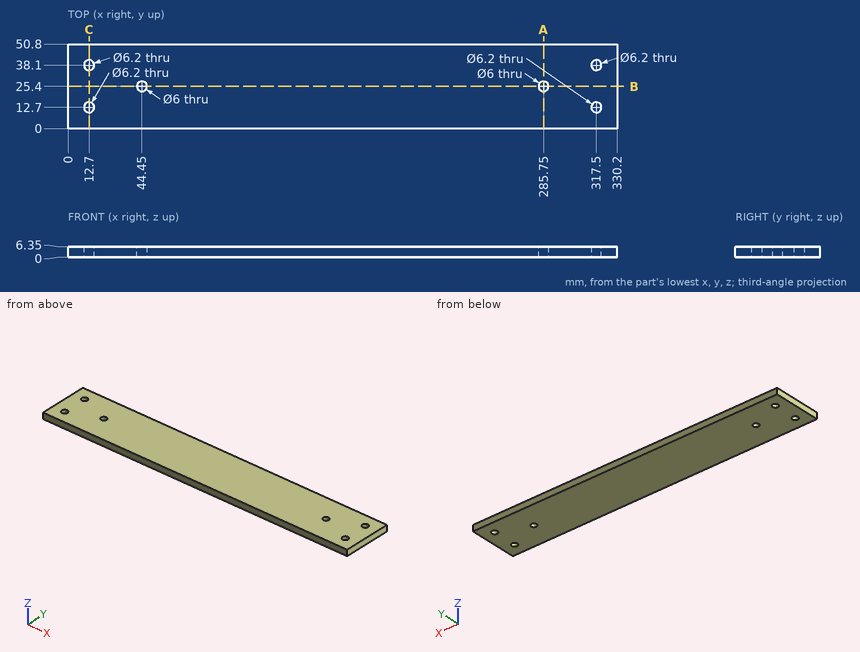
Input: dimensioned drawing with shaded views. Units: mm. Origin: part minimum x, y, z. Coordinates: 2 decimals unless noted, no trailing zeros. Order: outer loops, then holes, each group sorted by start corner. A loop starts at its lowest first (then second) coordinate and runs counter-clockwise, first axis right, second up.
Item 1: Section query C-C (x = 12.7). Output: boundary loops of the cut face in (y, z).
Answer:
outline: (0, 0) - (9.6, 0) - (9.6, 6.35) - (0, 6.35) - close; (15.8, 0) - (35, 0) - (35, 6.35) - (15.8, 6.35) - close; (41.2, 0) - (50.8, 0) - (50.8, 6.35) - (41.2, 6.35) - close
Item 2: Section query A-A (x = 285.75). Output: boundary loops of the cut face in (y, z), then the cut area to 3 significant figures.
Answer:
outline: (0, 0) - (22.4, 0) - (22.4, 6.35) - (0, 6.35) - close; (28.4, 0) - (50.8, 0) - (50.8, 6.35) - (28.4, 6.35) - close
area: 284 mm2
Item 3: Material intervals for line 1 along Y through (x, z) = (12.7, 3.5); line 2 along X through (y, z) = (10.5, 2.75); line 3 along X through (y, z) = (12, 4.75), sorted ascending.
Answer:
line 1: y = 0 to 9.6, 15.8 to 35, 41.2 to 50.8
line 2: x = 0 to 10.52, 14.88 to 315.32, 319.68 to 330.2
line 3: x = 0 to 9.68, 15.72 to 314.48, 320.52 to 330.2
Item 4: Section query B-B (y = 25.4). Output: boundary loops of the cut face in (x, z), then the cut area to 3 significant figures.
Answer:
outline: (0, 0) - (41.45, 0) - (41.45, 6.35) - (0, 6.35) - close; (47.45, 0) - (282.75, 0) - (282.75, 6.35) - (47.45, 6.35) - close; (288.75, 0) - (330.2, 0) - (330.2, 6.35) - (288.75, 6.35) - close
area: 2,020 mm2
